For this review, take the finished solid that the model builds, in its own axes (mm). A direction names the side the tool comes from. Give positions to 0.01 mm unless a question says otherwise; leave off trailing zeros. Loops run counter-clockwise (first coordinate to the right, second up) from the corner with the lowest first, then second, coordinate; pieces in that order, holes last. Notation, with made-up numbers: (-17, 35.5) -> (10, 35.5) arc R21 ccw to (10, 53.5) -> close; hole circle Ø7 at (-14.5, 27). An arc over 180 degrees is marked (long way). Answer as CSV lines item,"result". Start each with the question number.
Item 1: Add section B-B on z = 16.5. State the section outline as (x, y) points, plus the area to 3 significant figures.
Item 2: Add section A-A on x = -10. State the section outline as (y, z) points.
Item 3: Clearance check with flat-ended pins moving along their axes: P1, Ø2, axis at y = -22.5, z = 7.5, coming from the +X side; P2, Ø1, axis at y = 33.5, z = 9.5, coming from the +X side. State where each tip first meets the part, or that it passes through.
Item 4: The part is to be moulded in two halves that separate along X. For faces 3 (the face through (-42.714, 7, 12)), 4 (the face through (4.29, 19.26, 12.32)), 5 (the face through (0, -33.861, 12)), 6 (the face through (-15.89, 19.24, 12.32)), say which applies: +X half, -X half, draft (parallel to the pull), parting line (faces both ways), or undercut.
Item 5: Machinability: for faces 1 (the face through (38.204, -29.584, 12.325)), 2 (the face through (-6, -10.562, 12)), which of the approach directions +Z, -Z, +X, -X, +Y, -Y give a long, thin tool a straight path to every point of the face, cutting with its end or side? Answer none if there is none.
Item 6: Add section D-D on x = 35.5. State the section outline as (y, z) points.
Item 7: For L1, parallel to X at y = 16, z = 20; L2, parallel to Y at x = -19, z = 11.75; L3, parallel to Y at x = 5, z = 6.5, list the stretches that pass through material, from the lowest coordinate up. Write a range as from..to.
Item 8: Add section C-C on y = 12. State the section outline as (x, z) points, plus the area to 3 significant figures.
```python
from build123d import *

# Parameters (mm, degrees)
F1_DEPTH = 25


with BuildPart() as f1:
    # F0 (on Top) → F1 (new body)
    with BuildSketch(Plane.XY):
        with BuildLine():
            Line((-14.105032, 19.571008), (-27.714499, 47.588757))
            ThreePointArc((-27.714499, 47.588757), (-36.374753, 44.836205), (-41.856635, 37.588757))
            ThreePointArc((-41.856635, 37.588757), (-42.498477, 35.125286), (-42.714499, 32.588757))
            Line((-42.714499, 32.588757), (-19.105032, 14.571008))
            Line((-19.105032, 14.571008), (-19.105032, 18.328404))
            Line((-19.105032, 18.328404), (-17.403816, 18.328404))
            ThreePointArc((-17.403816, 18.328404), (-15.867562, 19.250056), (-14.105032, 19.571008))
        make_face()
        Polygon((27.714499, 47.588757), (-27.714499, 47.588757), (-14.105032, 19.571008), (2.551774, 19.571008), align=None)
        with BuildLine():
            ThreePointArc((42.714499, 32.588757), (38.321101, 43.195358), (27.714499, 47.588757))
            Line((27.714499, 47.588757), (2.551774, 19.571008))
            ThreePointArc((2.551774, 19.571008), (4.314304, 19.250056), (5.850558, 18.328404))
            Line((5.850558, 18.328404), (7.551774, 18.328404))
            Line((7.551774, 18.328404), (7.551774, 14.571008))
            Line((7.551774, 14.571008), (42.714499, 32.588757))
        make_face()
        Polygon((42.714499, -18.860948), (42.714499, 32.588757), (7.551774, 14.571008), (7.551774, -5.56213), align=None)
        Polygon((-19.105032, 14.571008), (-42.714499, 32.588757), (-42.714499, -18.860948), (-19.105032, -5.56213), align=None)
        with BuildLine():
            ThreePointArc((27.714499, -33.860948), (38.321101, -29.46755), (42.714499, -18.860948))
            Line((42.714499, -18.860948), (7.551774, -5.56213))
            Line((7.551774, -5.56213), (7.551774, -10.56213))
            Line((7.551774, -10.56213), (2.551774, -10.56213))
            Line((2.551774, -10.56213), (27.714499, -33.860948))
        make_face()
        with BuildLine():
            Line((-19.105032, -5.56213), (-42.714499, -18.860948))
            ThreePointArc((-42.714499, -18.860948), (-38.321101, -29.46755), (-27.714499, -33.860948))
            Line((-27.714499, -33.860948), (-14.105032, -10.56213))
            Line((-14.105032, -10.56213), (-19.105032, -10.56213))
            Line((-19.105032, -10.56213), (-19.105032, -5.56213))
        make_face()
        Polygon((-27.714499, -33.860948), (27.714499, -33.860948), (2.551774, -10.56213), (-14.105032, -10.56213), align=None)
    extrude(amount=F1_DEPTH)


solid = f1.part
```
Computed values:
1,outline,"(-42.71, -18.86) arc R15 ccw to (-27.71, -33.86) -> (27.71, -33.86) arc R15 ccw to (42.71, -18.86) -> (42.71, 32.59) arc R15 ccw to (27.71, 47.59) -> (-27.71, 47.59) arc R15 ccw to (-41.86, 37.59) arc R15 ccw to (-42.71, 32.59) -> close; hole (-19.11, -10.56) -> (7.55, -10.56) -> (7.55, 18.33) -> (5.85, 18.33) arc R5 ccw to (2.55, 19.57) -> (-14.11, 19.57) arc R5 ccw to (-17.4, 18.33) -> (-19.11, 18.33) -> close"
1,area,"5,970 mm²"
2,outline,"(-33.86, 0) -> (-10.56, 0) -> (-10.56, 25) -> (-33.86, 25) -> close; (19.57, 0) -> (47.59, 0) -> (47.59, 25) -> (19.57, 25) -> close"
3,P1,"x = 42.48"
3,P2,"x = 42.71"
4,face 3,"-X half"
4,face 4,"undercut"
4,face 5,"draft"
4,face 6,"undercut"
5,face 1,"+Z, -Z, +X, -Y"
5,face 2,"+Z, -Z"
6,outline,"(-31.68, 0) -> (45.41, 0) -> (45.41, 25) -> (-31.68, 25) -> close"
7,L1,"-42.71..-19.11, 7.55..42.71"
7,L2,"-33.86..-10.56, 18.33..47.59"
7,L3,"-33.86..-10.56, 18.93..47.59"
8,outline,"(-42.71, 0) -> (-19.11, 0) -> (-19.11, 25) -> (-42.71, 25) -> close; (7.55, 0) -> (42.71, 0) -> (42.71, 25) -> (7.55, 25) -> close"
8,area,"1,470 mm²"
